from build123d import *

# Parameters (mm, degrees)
F1_DEPTH  = 10
F2_DEPTH  = 150
F3_W      = 10
F3_H      = 70
F4_DEPTH  = 25
F5_R      = 10
F8_W      = 10
F8_H      = 70
F9_DEPTH  = 25
F7_W      = 10
F7_H      = 70
F10_DEPTH = 25
F6_W      = 10
F6_H      = 70
F11_DEPTH = 25


with BuildPart() as f1:
    # F0 (on Top) → F1 (new body)
    with BuildSketch(Plane.XY):
        Polygon((28.9362690725, 80.0640511845), (-149.8727713071, 80.0640511845), (-189.6601299418, 40.2766925498), (-189.6601299418, -138.3464388432), (-148.9716956383, -179.0348731467), (29.644071613, -179.0348731467), (69.624703376, -139.2548863311), (69.624703376, 39.375616881), align=None)
        Polygon((-184.6601299418, 38.205624738), (-147.8017034952, 75.0640511845), (26.8652012606, 75.0640511845), (64.624703376, 37.3045490692), (64.624703376, -137.1764467001), (27.5803679428, -174.0348731467), (-146.9006278264, -174.0348731467), (-184.6601299418, -136.2753710313), align=None, mode=Mode.SUBTRACT)
        Polygon((26.8652012606, 75.0640511845), (-147.8017034952, 75.0640511845), (-184.6601299418, 38.205624738), (-184.6601299418, -136.2753710313), (-146.9006278264, -174.0348731467), (27.5803679428, -174.0348731467), (64.624703376, -137.1764467001), (64.624703376, 37.3045490692), align=None)
    extrude(amount=F1_DEPTH)

    # F0 (on Top) → F2 (join)
    with BuildSketch(Plane.XY):
        Polygon((28.9362690725, 80.0640511845), (-149.8727713071, 80.0640511845), (-189.6601299418, 40.2766925498), (-189.6601299418, -138.3464388432), (-148.9716956383, -179.0348731467), (29.644071613, -179.0348731467), (69.624703376, -139.2548863311), (69.624703376, 39.375616881), align=None)
        Polygon((-184.6601299418, 38.205624738), (-147.8017034952, 75.0640511845), (26.8652012606, 75.0640511845), (64.624703376, 37.3045490692), (64.624703376, -137.1764467001), (27.5803679428, -174.0348731467), (-146.9006278264, -174.0348731467), (-184.6601299418, -136.2753710313), align=None, mode=Mode.SUBTRACT)
    extrude(amount=-F2_DEPTH)

    # F3 (on face) → F4 (cut)
    with BuildSketch(Plane(origin=(-164.0032843925, -164.0032843925, 0), x_dir=(0.7071067812, -0.7071067812, 0), z_dir=(-0.7071067812, -0.7071067812, 0))):
        with Locations((-7.5131911317, -115)):
            Rectangle(F3_W, F3_H)
    extrude(amount=-F4_DEPTH, mode=Mode.SUBTRACT)

    # F5
    f5_edges = [f1.edges().sort_by_distance(p)[0] for p in [
        (-60.468251, 80.064051, 10),
        (-169.766451, 60.170372, 10),
        (-189.66013, -49.034873, 10),
        (-169.315913, -158.690656, 10),
        (-59.663812, -179.034873, 10),
        (49.634387, -159.14488, 10),
        (69.624703, -49.939635, 10),
        (49.280486, 59.719834, 10),
    ]]
    fillet(f5_edges, radius=F5_R)

    # F8 (on face) → F9 (cut)
    with BuildSketch(Plane(origin=(-114.9684112458, 114.9684112458, 0), x_dir=(-0.7071067812, -0.7071067812, 0), z_dir=(-0.7071067812, 0.7071067812, 0))):
        with Locations((77.4961304807, -115)):
            Rectangle(F8_W, F8_H)
    extrude(amount=-F9_DEPTH, mode=Mode.SUBTRACT)

    # F7 (on face) → F10 (cut)
    with BuildSketch(Plane(origin=(54.5001601285, 54.5001601285, 0), x_dir=(-0.7071067812, 0.7071067812, 0), z_dir=(0.7071067812, 0.7071067812, 0))):
        with Locations((7.3817336266, -115)):
            Rectangle(F7_W, F7_H)
    extrude(amount=-F10_DEPTH, mode=Mode.SUBTRACT)

    # F6 (on face) → F11 (cut)
    with BuildSketch(Plane(origin=(104.2637675873, -104.7896601235, 0), x_dir=(0.7088833284, 0.7053257593, 0), z_dir=(0.7053257593, -0.7088833284, 0))):
        with Locations((-77.0639933351, -115)):
            Rectangle(F6_W, F6_H)
    extrude(amount=-F11_DEPTH, mode=Mode.SUBTRACT)


solid = f1.part
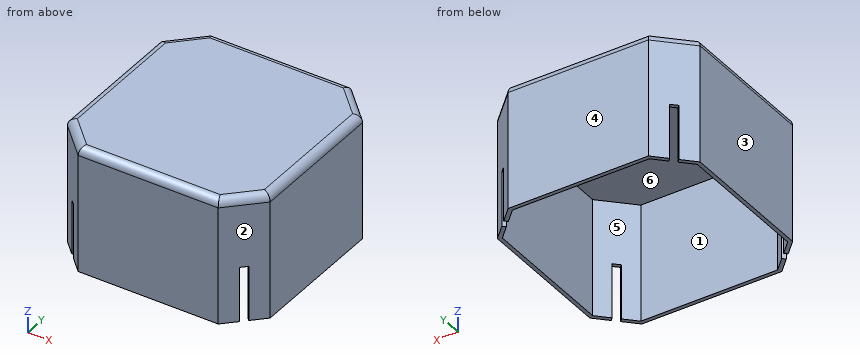
Read the model definition and answer for the solid it produces. Units are mm, in the model's axes. Face numbers are marked on the shaded views. A direction names the side the tool comes from. Coordinates: 2 decimals unless noted, no trailing zeros. Write each loop counter-clockwise with the first axis right and the second up, starting at its lowest first coordinate (ties: lowest second). Pieces come first, ordered by that corner, then holes. Notation, with made-up numbers: (48, 2) -> (78, 2) arc R21 cw to (78, 23) -> close; hole circle Ø11 at (52, -16). An arc over 180 degrees is marked (long way). Return JSON: item names as keys, results as strings.
(1) For a pull along X with two mould halves and no side action, classify the marked faces 3, 4, 5 and 6 as pulls with the +X half, pulls with the -X half, needs draft (parallel to the pull), parting line crosses it, or undercut.
Answers below:
{"face 3": "pulls with the -X half", "face 4": "needs draft", "face 5": "undercut", "face 6": "undercut"}
(2) Each of these flat-tipped pins is pushed along its axis until it touches: P1, Ø5.5, axis at x = 46.5, y = 57, coming from the -Z side; P2, Ø12, axis at y = 54, z = -12, coming from the -X side; P3, Ø1, axis at x = -72, y = 6, coming from the -Z side. Where does it stop, or does it pass through?
Answers below:
{"P1": "z = -80", "P2": "x = -181.94", "P3": "z = 0"}
(3) The part is cut by section D-D on y = -94. Give the vertices of the cut face in (x, z).
Answers below:
{"outline": "(-189.66, -150) -> (-184.66, -150) -> (-184.66, 0) -> (64.62, 0) -> (64.62, -150) -> (69.62, -150) -> (69.62, 0) arc R10 ccw to (59.62, 10) -> (-179.66, 10) arc R10 ccw to (-189.66, 0) -> close"}
(4) The part is cut by section A-A on z = -132. State how many separate pieces and enclosed holes the cut face has, then the cut area to 3 significant figures.
Answers below:
{"separate pieces": "4", "enclosed holes": "0", "area": "4,430 mm^2"}
(5) The part is cut by section B-B on z = -31.5. Give the vertices of the cut face in (x, y).
Answers below:
{"outline": "(-189.66, -138.35) -> (-148.97, -179.03) -> (29.64, -179.03) -> (69.62, -139.25) -> (69.62, 39.38) -> (28.94, 80.06) -> (-149.87, 80.06) -> (-189.66, 40.28) -> close; hole (-184.66, -136.28) -> (-146.9, -174.03) -> (27.58, -174.03) -> (64.62, -137.18) -> (64.62, 37.3) -> (26.87, 75.06) -> (-147.8, 75.06) -> (-184.66, 38.21) -> close"}
(6) Which of the six approach directions +Z, -Z, +X, -X, +Y, -Y give full straight-line access (tool end or side, diameter ignored) to the marked faces 1 and 2?
Answers below:
{"face 1": "-Z", "face 2": "+Z, -Z, +X, -Y"}
(7) The part is cut by section C-C on x = -133.5. Give the vertices of the cut face in (y, z).
Answers below:
{"outline": "(-179.03, -150) -> (-174.03, -150) -> (-174.03, 0) -> (75.06, 0) -> (75.06, -150) -> (80.06, -150) -> (80.06, 0) arc R10 ccw to (70.06, 10) -> (-169.03, 10) arc R10 ccw to (-179.03, 0) -> close"}
(8) Consider line 1 along X through (y, z) = (17, -115); line 2 along Y through (x, z) = (-75.5, -33.5); line 3 along Z through (x, y) = (12.5, -80). Determine where each line is inside the solid, lowest interval first. Write a range as from..to.
Answers below:
{"line 1": "-189.66..-184.66, 64.62..69.62", "line 2": "-179.03..-174.03, 75.06..80.06", "line 3": "0..10"}
